Design review of the part shown in the three views and the two pictorial views. Dimensions are in mm from the part's minimum x, y and z. A direction names the side the tool comes from. Give positions to 0.01 mm unless a question says otherwise; leave off trailing zeros. Order: outer loops, then holes, each group sorted by start corner. A loop starts at its lowest first (then second) coordinate and runs counter-clockwise, first axis right, second up. Notation, with made-up numbers: (23, 84) -> (62, 84) arc R24 ccw to (62, 120) -> close; hole circle Ø9 at (63.25, -27.5). An arc over 180 degrees is marked (long way). Use one line per item in the form item = value.
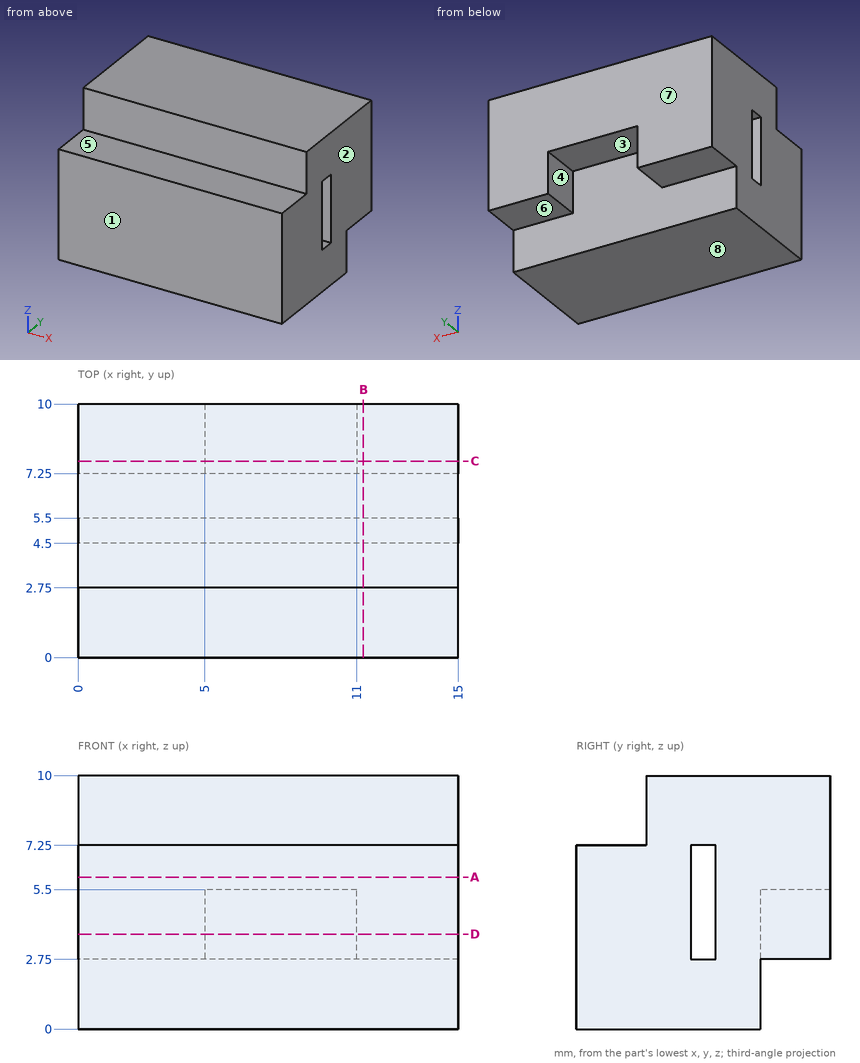
1. For pin 1 Ø1.4 at (x, y) = (6, 1) entering from +Z; pin 2 Ø3 at (x, y) = (13.5, 9) entering from -Z, all flat-tipped, find the tip position at first contact; note any pin that passes through.
Values:
pin_1 = 7.25
pin_2 = 2.75
2. Add section C-C on y = 7.75. Give the boundary of the cut face in (x, z).
Values:
outline = (0, 2.75) -> (5, 2.75) -> (5, 5.5) -> (11, 5.5) -> (11, 2.75) -> (15, 2.75) -> (15, 10) -> (0, 10) -> close
3. Add section D-D on z = 3.75. Give the boundary of the cut face in (x, y), then the cut area to 4 significant figures.
Values:
outline = (0, 0) -> (15, 0) -> (15, 4.5) -> (0, 4.5) -> close; (0, 5.5) -> (15, 5.5) -> (15, 10) -> (11, 10) -> (11, 7.25) -> (5, 7.25) -> (5, 10) -> (0, 10) -> close
area = 118.5 mm^2
4. Tool access review of the marked faces 4, 5, 6, 7 and 8: name each direction out of +Z, -Z, +X, -X, +Y, -Y from which nothing blocks a thin tool from reaching the whole face with its end or side.
Values:
face_4 = -Z, +Y
face_5 = +Z, +X, -X, -Y
face_6 = -Z, +X, -X, +Y
face_7 = +Z, -Z, +X, -X, +Y
face_8 = -Z, +X, -X, +Y, -Y
5. The part is to be moulded in two halves that separate along X. For the marked faces 1, 2 and 3, say which applies: +X half, -X half, draft (parallel to the pull), parting line (faces both ways), or undercut.
Values:
face_1 = draft
face_2 = +X half
face_3 = undercut
6. For L1, parallel to X at y = 9, z = 3; L2, parallel to Z at x = 2.75, y = 4.75; L3, parallel to Y at x = 10, z = 3.25, list the stretches that pass through material, from the lowest coordinate up.
Values:
L1 = 0 to 5, 11 to 15
L2 = 0 to 2.75, 7.25 to 10
L3 = 0 to 4.5, 5.5 to 7.25
7. Add section A-A on z = 6. Give the boundary of the cut face in (x, y), then the cut area to 3 significant figures.
Values:
outline = (0, 0) -> (15, 0) -> (15, 4.5) -> (0, 4.5) -> close; (0, 5.5) -> (15, 5.5) -> (15, 10) -> (0, 10) -> close
area = 135 mm^2
8. Add section B-B on x = 11.25. Give the boundary of the cut face in (y, z).
Values:
outline = (0, 0) -> (7.25, 0) -> (7.25, 2.75) -> (10, 2.75) -> (10, 10) -> (2.75, 10) -> (2.75, 7.25) -> (0, 7.25) -> close; hole (4.5, 2.75) -> (5.5, 2.75) -> (5.5, 7.25) -> (4.5, 7.25) -> close
